Design review of the part built by this model. Coordinates are the model's own, in mm. Round coordinates to 2 decimals unless told otherwise and drop trailing zeros. Loops run counter-clockwise (first coordinate to the right, second up) from the corner with the lowest first, then second, coordinate; pieces in that order, holes last. Notation, with made-up numbers: (45, 22) - (82, 22) arc R22 cw to (82, 39) - close; hole circle Ø4 at (72.5, -33). An arc over 180 degrees is marked (long way). One line per question, with ' | ' between items. Start each with the question number.
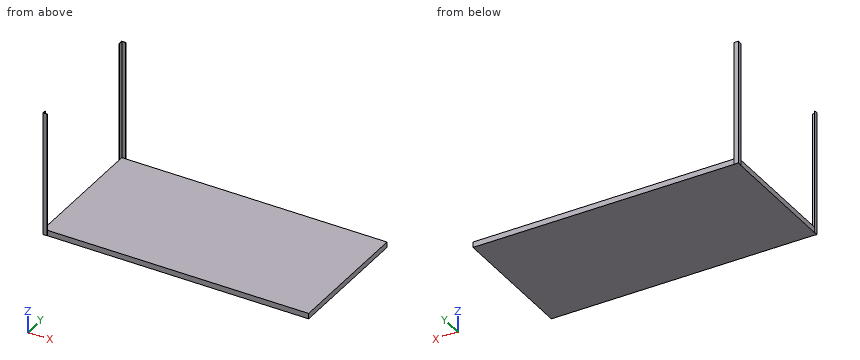
from build123d import *

# Parameters (mm, degrees)
F0_W     = 2438.4
F0_H     = 1219.2
F1_DEPTH = 50.8
F3_DEPTH = 1143


with BuildPart() as f1:
    # F0 (on Top) → F1 (new body)
    with BuildSketch(Plane.XY):
        Rectangle(F0_W, F0_H)
    extrude(amount=F1_DEPTH)

    # F2 (on face) → F3 (join)
    with BuildSketch(Plane(origin=(0, 0, 0), x_dir=(1, 0, 0), z_dir=(0, 0, -1))):
        Polygon((-1183.64, 612.14), (-1221.74, 612.14), (-1221.74, 574.04), (-1219.2, 574.04), (-1219.2, 609.6), (-1183.64, 609.6), align=None)
    extrude(amount=-F3_DEPTH)

    # F4: F1 across plane


with BuildPart() as f1_1:
    add(f1.part)
    add(f1.part.mirror(Plane.XZ))


solid = f1_1.part
1. Take a section at A-A, the plane z = 569. Give the boundary of the cut face in (x, y).
2. Take a section at C-C, the plane y = -53. Give the boundary of the cut face in (x, z).
3. Take a section at B-B, the plane x = -851.5. Give the boundary of the cut face in (y, z).
4. Clearance check with flat-ended pins moving along their axes: P1, Ø5, axis at x = -803.5, y = -204, coming from the +Z side; P2, Ø18, axis at y = -584, z = 481.5, coming from the +X side; P3, Ø2, axis at y = 610.5, z = 838.5, coming from the +X side. State where each tip first meets the part, or that it passes through.
5. To check wall thickness, follow line 1 along Z through (x, y) = (802, 140). State the ranges of the line that lie inside material, in increasing order.
Answer list:
1) outline: (-1221.74, -612.14) - (-1183.64, -612.14) - (-1183.64, -609.6) - (-1219.2, -609.6) - (-1219.2, -574.04) - (-1221.74, -574.04) - close; (-1221.74, 574.04) - (-1219.2, 574.04) - (-1219.2, 609.6) - (-1183.64, 609.6) - (-1183.64, 612.14) - (-1221.74, 612.14) - close
2) outline: (-1219.2, 0) - (1219.2, 0) - (1219.2, 50.8) - (-1219.2, 50.8) - close
3) outline: (-609.6, 0) - (609.6, 0) - (609.6, 50.8) - (-609.6, 50.8) - close
4) P1: stops at z = 50.8 | P2: stops at x = -1219.2 | P3: stops at x = -1183.64
5) line 1: z = 0 to 50.8
